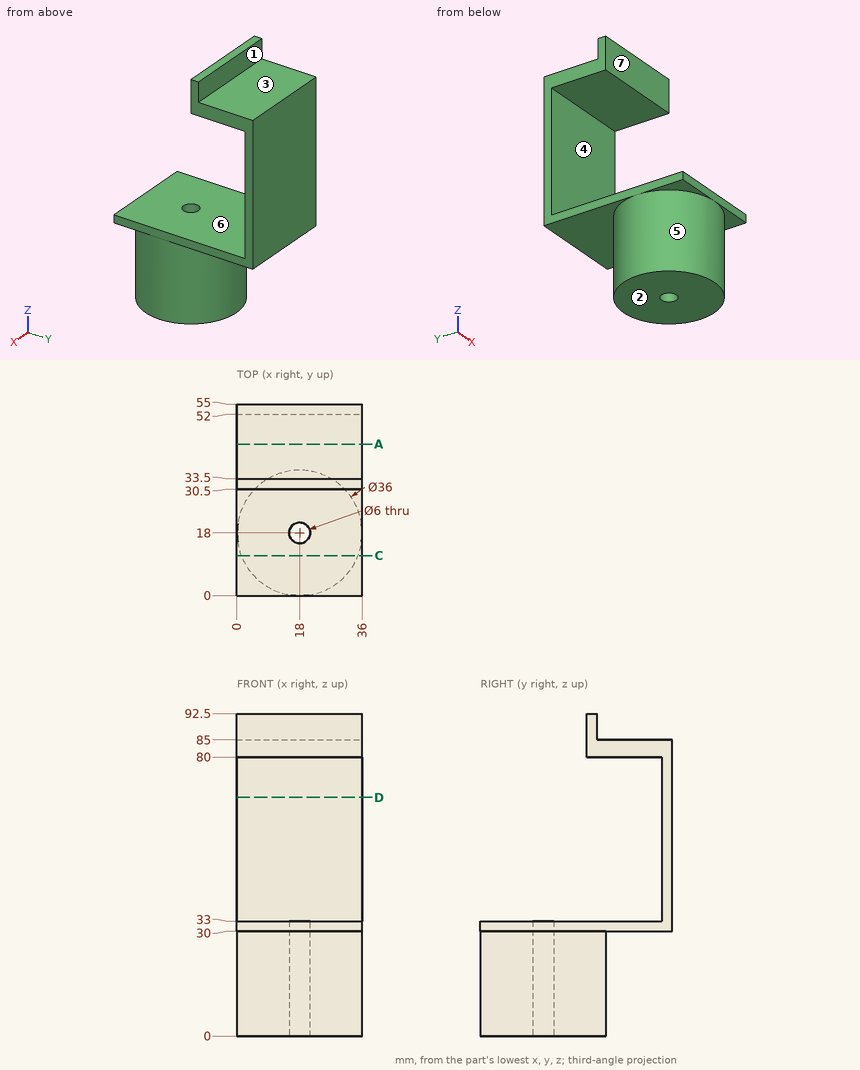
Part print with two shaded views. Sizes in mm from the minimum x, y, z corner. A direction names the side the tool comes from. Round coordinates to 2 decimals unless told otherwise and drop trailing zeros. Write each loop counter-clockwise with the first axis right and the second up, starting at its lowest first coordinate (ties: lowest second). Pieces come first, ordered by that corner, then holes. Notation, with made-up numbers: M -17,61 L -13,61 A10 cw -13,78 Z; hole C -35.5,82.5 d5. An arc over 180 degrees is marked long. Answer as CSV lines item,"result". Start each with the question number.
1) Mould opens along Z. For the marked faces 1, 2, 3 and 4 say: +Z half, -Z half, draft (parallel to the pull), parting line (faces both ways), or undercut.
2) Band-saw the part on A-A (y = 43.5). List the corners of the cut face in (x, z), then the cut area to 3 significant figures.
3) Drill centre lines: L1, parallel to Y at x = 18, z = 26; L2, parallel to Z at x = 25.5, y = 38; L3, parallel to Z at x = 11, y = 26.5. Where is each one in solid material? Low to high.
4) Drop flat-ended pins along their axis: pin 1 (4 mm diameter, centred on x = 19, z = 88.5, fed in from -Y); pin 2 (18 mm diameter, centred on x = 13, y = 27.5, fed in from +Z); pin 3 (1.5 mm diameter, centred on x = 25, y = 23, fed in from +Z); pin 4 (5 mm diameter, centred on x = 12, z = 26, fed in from +Y). Give the stop position or say it passes through.
5) Band-saw the part on C-C (y = 11.5). List the corners of the cut face in (x, z), then the cut area to 3 significant figures.
6) Which spindle directions (+Z, -Z, +X, -X, +Y, -Y) get a long thin tool onto all of the face, cutting with end or side? Do the marked faces 5, 6 and 7. Say none if no direction does.
7) Band-saw the part on D-D (z = 68.5). List the corners of the cut face in (x, y), then the cut area to 3 significant figures.
Worked out:
1,face 1,"draft"
1,face 2,"-Z half"
1,face 3,"+Z half"
1,face 4,"undercut"
2,outline,"M 0,30 L 36,30 L 36,33 L 0,33 Z; M 0,80 L 36,80 L 36,85 L 0,85 Z"
2,area,"288 mm²"
3,L1,"0 to 15, 21 to 36"
3,L2,"30 to 33, 80 to 85"
3,L3,"0 to 33"
4,pin 1,"y = 30.5"
4,pin 2,"z = 92.5"
4,pin 3,"z = 33"
4,pin 4,"y = 35.66"
5,outline,"M 0,30 L 1.21,30 L 1.21,0 L 34.79,0 L 34.79,30 L 36,30 L 36,33 L 0,33 Z"
5,area,"1,120 mm²"
6,face 5,"-Z"
6,face 6,"+X, -X, -Y"
6,face 7,"+Z, +X, -X, -Y"
7,outline,"M 0,52 L 36,52 L 36,55 L 0,55 Z"
7,area,"108 mm²"
